Geometry: final body of the model. Coordinates: model frame, mm. Round coordinates to 2 decimals unless told otherwise and drop trailing zeros. Order: outer loops, then holes, each group sorted by start corner. A loop starts at its lowest first (then second) coordinate and runs counter-clockwise, first axis right, second up. Notation, with made-up numbers: M 6,-26.75 L 14,-26.75 A16 ccw 14,-12.75 Z; hole C 79,38 d5. An arc over 180 degrees is marked long. Return JSON: item names as keys, results as strings. Group by question number.
Q1. Cut plane A-A on z = 0. Output: boundary loops of the cut face in (x, y), and give its area (3 significant figures).
Q2. Mould query, pull axis Y, two halves, no side actions, for faces 1 (the face through (7.222, -0.86, -3.874)), 2 (the face through (6.16, -1.89, -1.45)), 3 (the face through (1.588, -4, 1)). Classes: released by +Y, released by -Y, zero draft, split by the parting line, or undercut.
Q3. Ray query, probe 1 along Z at (x, y) = (8.25, 0); probe 2 along Z at (x, y) = (5.5, -0.5); probe 3 along X at (y, z) = (4, 0.5). Return the intervals inside material, ascending.
Q4. Cut plane C-C on x = 9. Output: boundary loops of the cut face in (y, z).
Q5. Contact query for flat-ended pins moving along their axis: pin 1 (4 mm diameter, centred on x = 9.5, y = -3.5, fed in from +Z); pin 2 (1.5 mm diameter, centred on x = 8, z = -2, fed in from +Y); pin 3 (2 mm diameter, centred on x = 9, y = -1, fed in from -Z); pin 4 (4 mm diameter, centred on y = 1, z = 1, fed in from -X). Output: stop coordinate, or through.
Q6. Cut plane D-D on y = -4.25. Output: boundary loops of the cut face in (x, z), and give its area (3 significant figures).
```python
from build123d import *

# Parameters (mm, degrees)
CHAMFER1_SIZE         = 0.5
CHAMFER1_SIZE2        = 0.288675135
CHAMFER1_PART_2_SIZE  = 0.5
CHAMFER1_PART_2_SIZE2 = 0.288675135


with BuildPart() as part:
    # Sketch1 → Revolve1 (revolve)
    with BuildSketch(Plane.XY):
        Polygon((0, 2.38125), (0, 5.55625), (1.5875, 5.55625), (1.5875, 3.96875), (12.7, 3.96875), (12.7, 2.38125), align=None)
    revolve(axis=Axis((0, 0, 0), (1, 0, 0)))

    # Chamfer1
    chamfer1_edges = [part.edges().sort_by_distance(p)[0] for p in [
        (12.7, -2.38125, 0),
    ]]
    chamfer1_side = [part.faces().sort_by_distance(p)[0] for p in [
        (6.35, -2.38125, 0),
    ]]
    chamfer(chamfer1_edges, length=CHAMFER1_SIZE, length2=CHAMFER1_SIZE2, reference=chamfer1_side[0])

    # Chamfer1 part 2
    chamfer1_part_2_edges = [part.edges().sort_by_distance(p)[0] for p in [
        (0, -2.38125, 0),
    ]]
    chamfer1_part_2_side = [part.faces().sort_by_distance(p)[0] for p in [
        (0, -2.538404482, 0),
    ]]
    chamfer(chamfer1_part_2_edges, length=CHAMFER1_PART_2_SIZE, length2=CHAMFER1_PART_2_SIZE2, reference=chamfer1_part_2_side[0])


solid = part.part
```
Result sheet:
{
 "1": {"outline": "M 0,-5.56 L 1.59,-5.56 L 1.59,-3.97 L 12.7,-3.97 L 12.7,-2.67 L 12.2,-2.38 L 0.29,-2.38 L 0,-2.88 Z; M 0,2.88 L 0.29,2.38 L 12.2,2.38 L 12.7,2.67 L 12.7,3.97 L 1.59,3.97 L 1.59,5.56 L 0,5.56 Z", "area": "45.1 mm²"},
 "2": {"face 1": "split by the parting line", "face 2": "undercut", "face 3": "zero draft"},
 "3": {"probe 1": "z = -3.97 to -2.38, 2.38 to 3.97", "probe 2": "z = -3.94 to -2.33, 2.33 to 3.94", "probe 3": "x = 0 to 1.59"},
 "4": {"outline": "C 0,0 d7.94; hole C 0,0 d4.76"},
 "5": {"pin 1": "stops at z = 3.67", "pin 2": "stops at y = 3.77", "pin 3": "stops at z = -3.97", "pin 4": "stops at x = 0"},
 "6": {"outline": "M 0,-3.58 L 1.59,-3.58 L 1.59,3.58 L 0,3.58 Z", "area": "11.4 mm²"}
}
